from build123d import *

# Parameters (mm, degrees)
F0_W     = 22
F0_H     = 22
F0_W_2   = 20
F0_H_2   = 20
F1_DEPTH = 12
F2_DEPTH = 1
F3_R     = 2


with BuildPart() as f1:
    # F0 (on Top) → F1 (new body)
    with BuildSketch(Plane.XY):
        Rectangle(F0_W, F0_H)
        Rectangle(F0_W_2, F0_H_2, mode=Mode.SUBTRACT)
    extrude(amount=F1_DEPTH)

    # F0 (on Top) → F2 (join)
    with BuildSketch(Plane.XY):
        Rectangle(F0_W, F0_H)
        Rectangle(F0_W_2, F0_H_2, mode=Mode.SUBTRACT)
        Rectangle(F0_W_2, F0_H_2)
    extrude(amount=-F2_DEPTH)

    # F3
    f3_edges = [f1.edges().sort_by_distance(p)[0] for p in [
        (-11, 11, 5.5),
        (-11, -11, 5.5),
        (11, 11, 5.5),
        (11, -11, 5.5),
    ]]
    fillet(f3_edges, radius=F3_R)


solid = f1.part
CAD build for the part. Positions are in the model's coordinates, mm. A direction names the side the tool comes from. Coordinates: 2 decimals unless noted, no trailing zeros. Write each loop counter-clockwise with the first axis right and the second up, starting at its lowest first coordinate (ties: lowest second). Pieces come first, ordered by that corner, then holes. Notation, with made-up numbers: (-31.75, 85) - (20.25, 85) arc R15 cw to (20.25, 107) - close; hole circle Ø1 at (-4.5, 83). An arc over 180 degrees is marked (long way). Use a Markdown table: item, result. Add a question column.
Item 1: Drill centre lines: L1, parallel to Y at x = -4.25, z = 2.75; L2, parallel to Z at x = 6, y = 9.25. Where is each one in solid material? Low to high. Write a range as from..to.
Item 2: 3-axis set-ups, long thin cutter, end or side, ignore diameter. For faces 4 (the face through (0, 0, 0)), 5 (the face through (10.43, 10.4, 5.41)): which of +Z, -Z, +X, -X, +Y, -Y reach the whole face in a straight line?
Item 3: Band-saw the part on A-A, the plane z = 4.75. Give the cut face in (x, y), and give its area (3 significant figures).
Item 4: Flat gauge pin, fed straight in: pin 1 (3 mm diameter, centred on x = 5.5, y = -3, fed in from +Z). Where does the tip first touch, or does it go through?
Item 5: Band-saw the part on B-B, the plane x = 7.25. Give the cut face in (y, z), and give its area (3 significant figures).
Item 6: Mould opens along X. For faces 1 (the face through (0, 10, 6)), 2 (the face through (10.43, -10.4, 5.59)), 3 (the face through (-10.43, -10.4, 5.59)) say: pulls with the +X half, pulls with the -X half, needs draft (parallel to the pull), parting line crosses it, or undercut.
Numbers:
| question | item | result |
|---|---|---|
| 1 | L1 | -11..-10, 10..11 |
| 1 | L2 | -1..0 |
| 2 | face 4 | +Z |
| 2 | face 5 | +Z, -Z, +X, +Y |
| 3 | outline | (-11, -9) arc R2 ccw to (-9, -11) - (9, -11) arc R2 ccw to (11, -9) - (11, 9) arc R2 ccw to (9, 11) - (-9, 11) arc R2 ccw to (-11, 9) - close; hole (-10, -10) - (10, -10) - (10, 10) - (-10, 10) - close |
| 3 | area | 80.6 mm2 |
| 4 | pin 1 | z = 0 |
| 5 | outline | (-11, -1) - (11, -1) - (11, 12) - (10, 12) - (10, 0) - (-10, 0) - (-10, 12) - (-11, 12) - close |
| 5 | area | 46.0 mm2 |
| 6 | face 1 | undercut |
| 6 | face 2 | pulls with the +X half |
| 6 | face 3 | pulls with the -X half |
